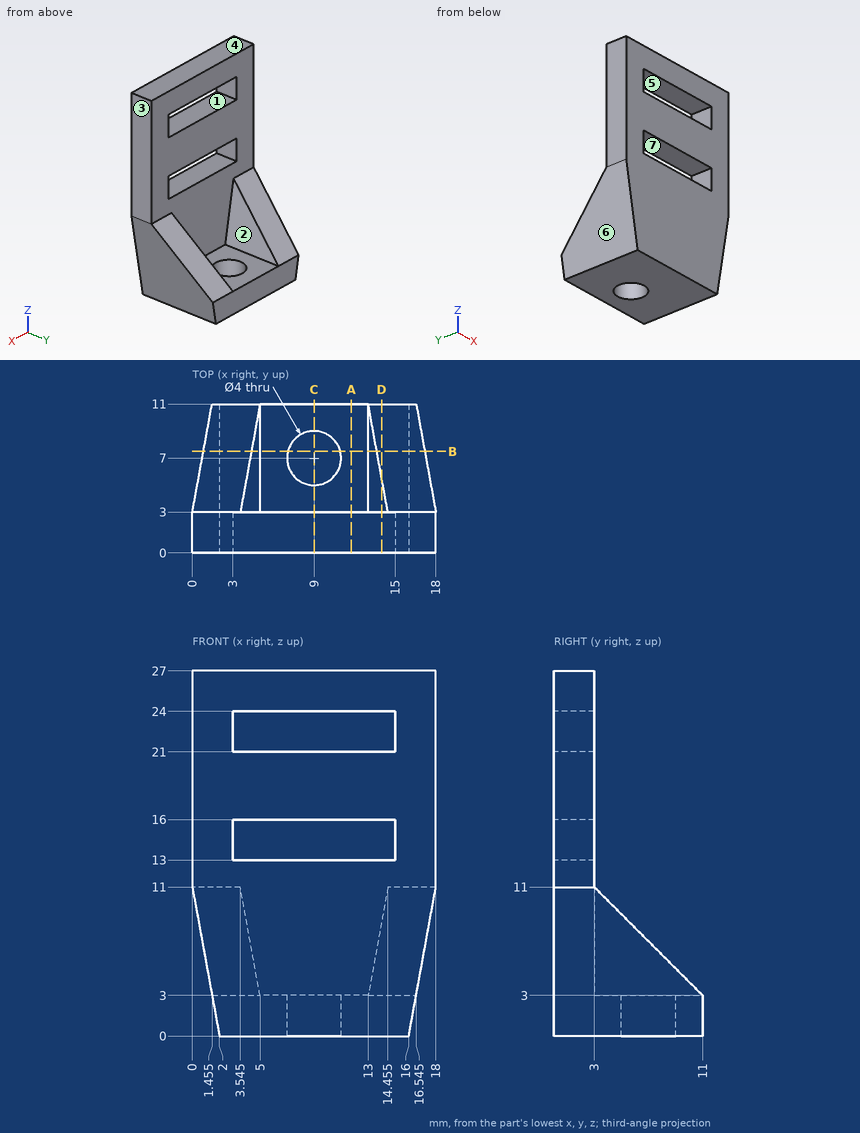
Part print with two shaded views. Sizes in mm from the minimum x, y, z corner. A direction names the side the tool comes from. Round coordinates to 2 decimals unless told otherwise and drop trailing zeros. Order: outer loops, then holes, each group sorted by start corner. A loop starts at its lowest first (then second) coordinate and runs counter-clockwise, first axis right, second up. Notation, with made-up numbers: (24, 86.5) - (79, 86.5) arc R9 ccw to (79, 97.5) - close; hole circle Ø2 at (73.25, 54.25). An arc over 180 degrees is marked (long way). Answer as CSV lines item,"result". Start each with the question number.
1. Saw through at D-D, the plane x = 14. Write the cut outline in (y, z).
2. Saw through at A-A, the plane x = 11.75. Write the cut outline in (y, z).
3. Pin check, flat tips, straight feed: pin 1 (8 mm diameter, centred on x = 8.5, z = 11, fed in from +Y); pin 2 (8 mm diameter, centred on x = 14, z = 11.5, fed in from +Y); pin 3 (6.5 mm diameter, centred on x = 9.5, y = 7.5, fed in from +Z). Stop position of each tip, or through.
4. Drill centre lines: L1, parallel to Z at x = 4.75, y = 2; L2, parallel to Y at x = 9, z = 1.15; L3, parallel to Y at x = 10.5, z = 1 (1 decimal). Where is each one in solid material? Low to high. Write a range as [from, to].
5. Saw through at C-C, the plane x = 9. Write the cut outline in (y, z).
6. Pull direction X, two halves, no side cores. Call the marked faces 4, 5, 6 and 7: +X half, -X half, draft (parallel to the pull), parting line (faces both ways), or undercut.
7. Tool access for the marked faces 1, 2 and 3: list every direction of +Z, -Z, +X, -X, +Y, -Y with a clear straight run to the whole face (end or side of a thin tool).
8. Saw through at B-B, the plane y = 7.5. Write the cut outline in (x, z).
Model answer:
1,outline,"(0, 0) - (11, 0) - (11, 3) - (5.5, 8.5) - (3, 8.5) - (3, 13) - (0, 13) - close; (0, 16) - (3, 16) - (3, 21) - (0, 21) - close; (0, 24) - (3, 24) - (3, 27) - (0, 27) - close"
2,outline,"(0, 0) - (11, 0) - (11, 3) - (3, 3) - (3, 13) - (0, 13) - close; (0, 16) - (3, 16) - (3, 21) - (0, 21) - close; (0, 24) - (3, 24) - (3, 27) - (0, 27) - close"
3,pin 1,"stops at y = 3"
3,pin 2,"stops at y = 6.5"
3,pin 3,"stops at z = 3"
4,L1,"z = [0, 13], [16, 21], [24, 27]"
4,L2,"y = [0, 5], [9, 11]"
4,L3,"y = [0, 5.7], [8.3, 11]"
5,outline,"(0, 0) - (5, 0) - (5, 3) - (3, 3) - (3, 13) - (0, 13) - close; (0, 16) - (3, 16) - (3, 21) - (0, 21) - close; (0, 24) - (3, 24) - (3, 27) - (0, 27) - close; (9, 0) - (11, 0) - (11, 3) - (9, 3) - close"
6,face 4,"draft"
6,face 5,"undercut"
6,face 6,"-X half"
6,face 7,"undercut"
7,face 1,"+Y, -Y"
7,face 2,"+Z, +Y"
7,face 3,"+Z, -Z, +X, +Y, -Y"
8,outline,"(0.82, 6.5) - (2, 0) - (7.06, 0) - (7.06, 3) - (5, 3) - (4.36, 6.5) - close; (10.94, 0) - (16, 0) - (17.18, 6.5) - (13.64, 6.5) - (13, 3) - (10.94, 3) - close"
